For this review, take the finished solid that the model builds, in its own axes (mm). Face numbers are marked on the shaded views. A direction names the side the tool comes from. Round coordinates to 2 decimals unless told otherwise and drop trailing zeros. Order: outer loops, then holes, each group sorted by start corner. A loop starts at its lowest first (then second) coordinate and runs counter-clockwise, first axis right, second up. Notation, with made-up numbers: (-14.75, 41) -> (40.25, 41) arc R23 cw to (40.25, 54) -> close; hole circle Ø8 at (15, -15.5). An arc over 180 degrees is marked (long way). Answer in a Markdown table with one row per item.
Autodesk Fusion 360 part; units mm, degrees
sketch "Sketch1" plane through (0, 0, 0) normal (0, 0, 1) x (1, 0, 0)
  line L0 (0, 0) -> (50, 0)
  line L1 (50, 0) -> (50, 50)
  line L2 (50, 50) -> (0, 50)
  line L3 (0, 50) -> (0, 0)
  dimension "d1" = 50
  dimension "d2" = 50
extrude "Extrude1" add sketch "Sketch1" along normal blind 5
sketch "Sketch2" plane through (0, 0, 5) normal (0, 0, 1) x (-1, 0, 0)
  line L0 (0, -50) -> (0, 0)
  line L1 (0, 0) -> (-50, 0)
  line L2 (-50, 0) -> (-50, -50)
  line L3 (-50, -50) -> (0, -50)
  circle A0 centre (-10, -40) radius 5
  circle A1 centre (-40, -40) radius 5
  dimension "d5" = 10
  dimension "d6" = 10
extrude "Extrude2" cut sketch "Sketch2" against normal blind 2 contours A0 | A1
sketch "Sketch3" plane through (0, 0, 3) normal (0, 0, 1) x (-1, 0, 0)
  circle A0 centre (-10, -40) radius 5
  circle A1 centre (-10, -40) radius 3
  circle A2 centre (-40, -40) radius 3
  dimension "d9" = 6
  dimension "d10" = 6
extrude "Extrude3" cut sketch "Sketch3" against normal blind 5 contours A1 | A2
sketch "Sketch4" plane through (0, 0, 0) normal (0, 0, -1) x (1, 0, 0)
  circle A0 centre (10, -40) radius 3
  circle A1 centre (40, -40) radius 3
  line L0 (0, 0) -> (0, -50)
  line L1 (0, -50) -> (50, -50)
  line L2 (50, -50) -> (50, 0)
  line L3 (50, 0) -> (0, 0)
  line L4 (0, 0) -> (10, 0)
  line L5 (10, 0) -> (10, -10)
  line L6 (10, -10) -> (0, -10)
  line L7 (0, -10) -> (0, 0)
  line L8 (50, 0) -> (40, 0)
  line L9 (40, 0) -> (40, -10)
  line L10 (40, -10) -> (50, -10)
  line L11 (50, -10) -> (50, 0)
  dimension "d13" = 10
  dimension "d14" = 10
  dimension "d15" = 10
  dimension "d16" = 10
extrude "Extrude4" add sketch "Sketch4" along normal blind 15 contours L0 L3 L4 L5 L6 L7 | L2 L3 L8 L9 L10 L11
sketch "Sketch5" plane through (50, 0, 0) normal (1, 0, 0) x (0, 1, 0)
  line L0 (10, 0) -> (50, 0)
  line L1 (50, 0) -> (50, 5)
  line L2 (50, 5) -> (0, 5)
  line L3 (0, 5) -> (0, -15)
  line L4 (0, -15) -> (10, -15)
  line L5 (10, -15) -> (10, 0)
  circle A0 centre (5, -10) radius 3.5
  dimension "d19" = 7
extrude "Extrude5" cut sketch "Sketch5" against normal blind 50 contours A0
sketch "Sketch6" plane through (0, 10, 0) normal (0, 1, 0) x (-1, 0, 0)
  line L0 (-40, 0) -> (-50, 0)
  line L1 (-50, 0) -> (-50, -15)
  line L2 (-50, -15) -> (-40, -15)
  line L3 (-40, -15) -> (-40, 0)
  line L4 (45, -6.5) -> (-55, -6.5)
  line L5 (-55, -6.5) -> (-55, -13.5)
  line L6 (-55, -13.5) -> (45, -13.5)
  line L7 (45, -13.5) -> (45, -6.5)
  line L8 (45, -6.5) -> (-55, -13.5) construction
  line L9 (-55, -6.5) -> (45, -13.5) construction
  point P0 (-5, -10)
  dimension "d22" = 100
  dimension "d23" = 7
extrude "Extrude6" cut sketch "Sketch6" against normal blind 5 contours L3 L4 L6 L7 | L1 L3 L4 L6 | L1 L4 L5 L6
sketch "Sketch7" plane through (50, 0, 0) normal (1, 0, 0) x (0, 1, 0)
  line L0 (5, -6.5) -> (10, -6.5)
  line L1 (10, -6.5) -> (10, 0)
  line L2 (10, 0) -> (50, 0)
  line L3 (50, 0) -> (50, 5)
  line L4 (50, 5) -> (0, 5)
  line L5 (0, 5) -> (0, -15)
  line L6 (0, -15) -> (10, -15)
  line L7 (10, -15) -> (10, -13.5)
  line L8 (10, -13.5) -> (5, -13.5)
  arc A0 (5, -6.5) -> (5, -13.5) centre (5, -10) ccw
  circle A1 centre (5, 2.5) radius 2.5
  dimension "d26" = 5
extrude "Extrude7" add sketch "Sketch7" along normal blind 5 contours A1
sketch "Sketch8" plane through (0, 0, 0) normal (-1, 0, 0) x (0, -1, 0)
  line L0 (-10, -6.5) -> (-5, -6.5)
  arc A0 (-5, -13.5) -> (-5, -6.5) centre (-5, -10) ccw
  line L1 (-5, -13.5) -> (-10, -13.5)
  line L2 (-10, -13.5) -> (-10, -15)
  line L3 (-10, -15) -> (0, -15)
  line L4 (0, -15) -> (0, 5)
  line L5 (0, 5) -> (-50, 5)
  line L6 (-50, 5) -> (-50, 0)
  line L7 (-50, 0) -> (-10, 0)
  line L8 (-10, 0) -> (-10, -6.5)
  circle A1 centre (-5, 2.5) radius 2.5
  dimension "d29" = 5
extrude "Extrude8" add sketch "Sketch8" along normal blind 5 contours A1
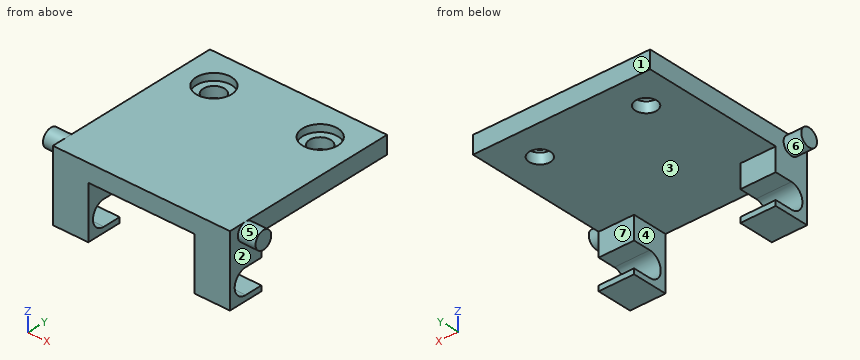
Q1. Take a section at C-C, the plane x = 49. Write out the cut boundary in (y, z).
Answer key:
| item | result |
|---|---|
| outline | (0, -15) -> (10, -15) -> (10, -13.5) -> (5, -13.5) arc R3.5 cw to (5, -6.5) -> (10, -6.5) -> (10, 0) -> (50, 0) -> (50, 5) -> (0, 5) -> close |
Q2. Take a section at D-D, the plane x = 38.5. Write out the cut boundary in (y, z).
Answer key:
| item | result |
|---|---|
| outline | (0, 0) -> (37.4, 0) -> (37.4, 3) -> (35.23, 3) -> (35.23, 5) -> (0, 5) -> close; (42.6, 0) -> (50, 0) -> (50, 5) -> (44.77, 5) -> (44.77, 3) -> (42.6, 3) -> close |
Q3. To check wall thickness, follow probe 1 along X at (y, z) = (40, 2); probe 2 along X at (y, z) = (40, 4.25); probe 3 along Y at (x, z) = (40, 2.2). State the ranges of each line that lie inside material, in increasing order.
Answer key:
| item | result |
|---|---|
| probe 1 | x = 0 to 7, 13 to 37, 43 to 50 |
| probe 2 | x = 0 to 5, 15 to 35, 45 to 50 |
| probe 3 | y = 0 to 37, 43 to 50 |
Q4. The part is to be moulded in two halves that separate along X. For the marked faces 1, 2 and 3, say which applies: +X half, -X half, draft (parallel to the pull), parting line (faces both ways), or undercut.
Answer key:
| item | result |
|---|---|
| face 1 | draft |
| face 2 | +X half |
| face 3 | undercut |
Q5. Clearance check with flat-ended pins moving along their axes: pin 1 Ø12 at (x, z) = (33.5, -1.5) entering from -Y; pin 2 Ø8 at (x, y) = (38, 17.5) entering from -Z; pin 3 Ø12 at (y, z) = (26.5, 2.5) entering from -X; pin 4 Ø0.8 at (x, z) = (6.5, -14) entering from +Y. State where each tip first meets the part, or that it passes through.
Answer key:
| item | result |
|---|---|
| pin 1 | stops at y = 0 |
| pin 2 | stops at z = 0 |
| pin 3 | stops at x = 0 |
| pin 4 | stops at y = 10 |
Q6. Take a section at B-B, the plane z = -10. Write out the cut boundary in (x, y), then the cut area to 3 significant figures.
Answer key:
| item | result |
|---|---|
| outline | (0, 0) -> (10, 0) -> (10, 1.5) -> (0, 1.5) -> close; (40, 0) -> (50, 0) -> (50, 1.5) -> (40, 1.5) -> close |
| area | 30.0 mm^2 |
Q7. Take a section at A-A, the plane y = 40. Write out the cut boundary in (x, z).
Answer key:
| item | result |
|---|---|
| outline | (0, 0) -> (7, 0) -> (7, 3) -> (5, 3) -> (5, 5) -> (0, 5) -> close; (13, 0) -> (37, 0) -> (37, 3) -> (35, 3) -> (35, 5) -> (15, 5) -> (15, 3) -> (13, 3) -> close; (43, 0) -> (50, 0) -> (50, 5) -> (45, 5) -> (45, 3) -> (43, 3) -> close |
Q8. Tool access review of the marked faces 4, 5, 6 and 7: name each direction out of +Z, -Z, +X, -X, +Y, -Y from which nothing blocks a thin tool from reaching the whole face with its end or side.
Answer key:
| item | result |
|---|---|
| face 4 | -Z, +Y, -Y |
| face 5 | +X |
| face 6 | -X |
| face 7 | -Z, +X, -X, +Y |
